```python
from build123d import *

# Parameters (mm, degrees)
SKETCH1_W               = 47.625
SKETCH1_H               = 22.225
BOSS_EXTRUDE1_DEPTH     = 23.8125
F_1_4_CLEARANCE_HOLE1_D = 6.7564
F_1_4_CLEARANCE_HOLE2_D = 6.7564
CHAMFER1_SIZE           = 1.524


with BuildPart() as part:
    # Sketch1 → Boss-Extrude1 (new, symmetric)
    with BuildSketch(Plane(origin=(0, 0, 0), x_dir=(0, 0, -1), z_dir=(1, 0, 0))):
        Rectangle(SKETCH1_W, SKETCH1_H)
    extrude(amount=BOSS_EXTRUDE1_DEPTH, both=True)

    # 1/4 Clearance Hole1 (through all)
    with Locations(Plane.XY.offset(23.8125)):
        with Locations((0, 0), (-15.875, 0), (15.875, 0)):
            Hole(F_1_4_CLEARANCE_HOLE1_D / 2)

    # 1/4 Clearance Hole2 (through all)
    with Locations(Plane(origin=(0, 11.1125, 0), x_dir=(1, 0, 0), z_dir=(0, 1, 0))):
        with Locations((-15.875, 0), (15.875, 0), (0, 0)):
            Hole(F_1_4_CLEARANCE_HOLE2_D / 2)

    # Chamfer1
    chamfer1_edges = [part.edges().sort_by_distance(p)[0] for p in [
        (23.8125, 0, -23.8125),
        (23.8125, 11.1125, 0),
        (23.8125, 0, 23.8125),
        (-23.8125, 11.1125, 0),
        (-23.8125, 0, -23.8125),
        (-23.8125, -11.1125, 0),
        (-23.8125, 0, 23.8125),
        (0, 11.1125, 23.8125),
        (0, 11.1125, -23.8125),
        (0, -11.1125, -23.8125),
        (0, -11.1125, 23.8125),
        (23.8125, -11.1125, 0),
    ]]
    chamfer(chamfer1_edges, length=CHAMFER1_SIZE)


solid = part.part
```
Geometry check sheet. Reference: the model listing, model coordinates, mm. Round coordinates to 2 decimals unless told otherwise and drop trailing zeros. Write each loop counter-clockwise with the first axis right and the second up, starting at its lowest first coordinate (ties: lowest second). Pieces come first, ordered by that corner, then holes. Notation, with made-up numbers: (-30, 70) -> (22, 70) arc R11 ccw to (22, 84) -> close; hole circle Ø6 at (86.25, -7). An arc over 180 degrees is marked (long way). Put each result on its own line as item: value.
1) Depth check by flat-ended pin: P1, Ø11, axis at x = -15.875, z = 0, coming from the -Y side; P2, Ø5.5, axis at x = 0, y = 0, coming from the -Z side. Enter the tip coordinate at first touch or a pass-through.
Recorded:
P1: stops at y = -11.11
P2: passes through
2) Thickness scan on probe 1 along X at (y, z) = (-0.25, 21); probe 2 along X at (y, z) = (2.75, -7); probe 3 along Y at (x, z) = (0, 5). Record the ranges inside material, lowest first. Write a range as from..to.
Recorded:
probe 1: x = -23.81..-19.24, -12.51..-3.37, 3.37..12.51, 19.24..23.81
probe 2: x = -23.81..-17.84, -13.91..-1.96, 1.96..13.91, 17.84..23.81
probe 3: y = -11.11..-3.38, 3.38..11.11
3) Release check for a two-part mould opening along Z. For faces 1 (the face through (-22.77, 10.05, 22.87)), 2 (the face through (0.3, 10.3, -23.1)), 3 (the face through (-18.996, 6.713, 1.294)), 4 (the face through (-3.222, 6.713, -1.015)) record: pulls with the +Z half, pulls with the -Z half, needs draft (parallel to the pull), parting line crosses it, or undercut.
Recorded:
face 1: pulls with the +Z half
face 2: pulls with the -Z half
face 3: undercut
face 4: undercut
4) Cross-section at C-C, the plane z = -19. Enter the section's corners in (x, y) (1 decimal), plus the area to 3 significant figures.
Recorded:
outline: (-23.8, -9.6) -> (-22.3, -11.1) -> (22.3, -11.1) -> (23.8, -9.6) -> (23.8, 9.6) -> (22.3, 11.1) -> (-22.3, 11.1) -> (-23.8, 9.6) -> close; hole circle Ø6.8 at (-15.9, 0); hole circle Ø6.8 at (0, 0); hole circle Ø6.8 at (15.9, 0)
area: 946 mm2
5) Cross-section at D-D, the plane y = 2. Give the number of separate pieces and of enclosed holes in the cut face, plus the area to 3 significant figures.
Recorded:
separate pieces: 4
enclosed holes: 0
area: 1,470 mm2
6) Cross-section at B-B, the plane y = -5. Enter the section's corners in (x, z) (1 decimal).
Recorded:
outline: (-23.8, -22.3) -> (-22.3, -23.8) -> (22.3, -23.8) -> (23.8, -22.3) -> (23.8, 22.3) -> (22.3, 23.8) -> (-22.3, 23.8) -> (-23.8, 22.3) -> close; hole circle Ø6.8 at (-15.9, 0); hole circle Ø6.8 at (0, 0); hole circle Ø6.8 at (15.9, 0)
7) Cross-section at A-A, the plane x = 0. Enter the section's corners in (y, z), plus the area to 3 significant figures.
Recorded:
outline: (-11.11, -22.29) -> (-9.59, -23.81) -> (-3.38, -23.81) -> (-3.38, -3.38) -> (-11.11, -3.38) -> close; (-11.11, 3.38) -> (-3.38, 3.38) -> (-3.38, 23.81) -> (-9.59, 23.81) -> (-11.11, 22.29) -> close; (3.38, -23.81) -> (9.59, -23.81) -> (11.11, -22.29) -> (11.11, -3.38) -> (3.38, -3.38) -> close; (3.38, 3.38) -> (11.11, 3.38) -> (11.11, 22.29) -> (9.59, 23.81) -> (3.38, 23.81) -> close
area: 628 mm2
